For this review, take the finished solid that the model builds, in its own axes (mm). Coordinates: 2 decimals unless noted, no trailing zeros. Loops run counter-clockwise (first coordinate to the right, second up) from the corner with the lowest first, then second, coordinate; pieces in that order, holes last.
1. Take a section at A-A, the plane y = -70. State the section outline as (x, z) points, then the cut area to 3 significant figures.
2. Take a section at C-C, the plane y = 0. State the section outline as (x, z) points, then the cut area to 3 significant figures.
3. Take a section at D-D, the plane z = 4.2. State the section outline as (x, y) points, then the cut area to 3 significant figures.
4. To check wall thickness, follow probe 1 along Y at (x, z) = (40, 3.6); probe 2 along Y at (x, z) = (0, 3.8); probe 3 along X at (y, z) = (-48.5, 0.35). State the ranges of each line that lie inside material, in increasing order.
5. Clearance check with flat-ended pins moving along their axes: P1, Ø3, axis at x = 16.5, z = 2.5, coming from the +Y side; P2, Ø3, axis at x = 25.5, z = 1, coming from the +Y side; P3, Ø1, axis at y = 8.5, z = 3, coming from the -X side. State where each tip first meets the part, or that it passes through.
6. Take a section at B-B, the plane x = -40. State the section outline as (y, z) points.
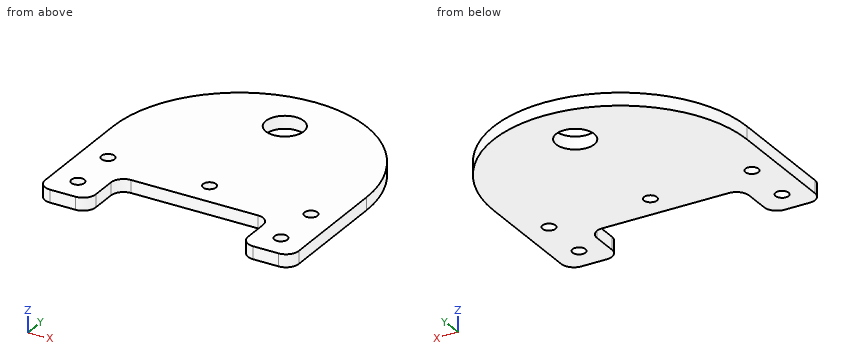
```python
from build123d import *

# Parameters (mm, degrees)
SKETCH_1_R      = 7.5
SKETCH_1_R_2    = 2.55
EXTRUDE_1_DEPTH = 5
SKETCH_2_W      = 20
SKETCH_2_H      = 20
SKETCH_2_R      = 2.55
EXTRUDE_2_DEPTH = 5
FILLET_1_R      = 5


with BuildPart() as part:
    # ｽｹｯﾁ1 → ﾎﾞｽ - 押し出し1 (new body)
    with BuildSketch(Plane.XY):
        with BuildLine():
            Line((-50, -60), (50, -60))
            Line((50, -60), (50, -30))
            ThreePointArc((50, -30), (0, 20), (-50, -30))
            Line((-50, -30), (-50, -60))
        make_face()
        Circle(SKETCH_1_R, mode=Mode.SUBTRACT)
        with Locations((-40, -50)):
            Circle(SKETCH_1_R_2, mode=Mode.SUBTRACT)
        with Locations((0, -50)):
            Circle(SKETCH_1_R_2, mode=Mode.SUBTRACT)
        with Locations((40, -50)):
            Circle(SKETCH_1_R_2, mode=Mode.SUBTRACT)
    extrude(amount=EXTRUDE_1_DEPTH)

    # ｽｹｯﾁ2 → ﾎﾞｽ - 押し出し2 (add)
    # profile 1 of 2: a face of its own
    with BuildSketch(Plane.XY.offset(5)):
        with Locations((-40, -70)):
            Rectangle(SKETCH_2_W, SKETCH_2_H)
        with Locations((-40, -70)):
            Circle(SKETCH_2_R, mode=Mode.SUBTRACT)
    # profile 2 of 2: a face of its own
    with BuildSketch(Plane.XY.offset(5)):
        with Locations((40, -70)):
            Rectangle(SKETCH_2_W, SKETCH_2_H)
        with Locations(Location((40, -70, 0), (0, 0, 180))):
            Circle(SKETCH_2_R, mode=Mode.SUBTRACT)
    extrude(amount=-EXTRUDE_2_DEPTH)

    # ﾌｨﾚｯﾄ1
    fillet_1_edges = [part.edges().sort_by_distance(p)[0] for p in [
        (-50, -80, 2.5),
        (-30, -60, 2.5),
        (-30, -80, 2.5),
        (30, -60, 2.5),
        (50, -80, 2.5),
        (30, -80, 2.5),
    ]]
    fillet(fillet_1_edges, radius=FILLET_1_R)


solid = part.part
```
Results list:
1. outline: (-50, 0) - (-42.55, 0) - (-42.55, 5) - (-50, 5) - close; (-37.45, 0) - (-30, 0) - (-30, 5) - (-37.45, 5) - close; (30, 0) - (37.45, 0) - (37.45, 5) - (30, 5) - close; (42.55, 0) - (50, 0) - (50, 5) - (42.55, 5) - close
1. area: 149 mm2
2. outline: (-40, 0) - (-7.5, 0) - (-7.5, 5) - (-40, 5) - close; (7.5, 0) - (40, 0) - (40, 5) - (7.5, 5) - close
2. area: 325 mm2
3. outline: (-50, -75) arc R5 ccw to (-45, -80) - (-35, -80) arc R5 ccw to (-30, -75) - (-30, -65) arc R5 cw to (-25, -60) - (25, -60) arc R5 cw to (30, -65) - (30, -75) arc R5 ccw to (35, -80) - (45, -80) arc R5 ccw to (50, -75) - (50, -30) arc R50 ccw to (-50, -30) - close; hole circle Ø5.1 at (-40, -70); hole circle Ø5.1 at (-40, -50); hole circle Ø15 at (0, 0); hole circle Ø5.1 at (0, -50); hole circle Ø5.1 at (40, -70); hole circle Ø5.1 at (40, -50)
3. area: 7,440 mm2
4. probe 1: y = -80 to -72.55, -67.45 to -52.55, -47.45 to 0
4. probe 2: y = -60 to -52.55, -47.45 to -7.5, 7.5 to 20
4. probe 3: x = -50 to -42.06, -37.94 to -2.06, 2.06 to 37.94, 42.06 to 50
5. P1: stops at y = 17.7
5. P2: stops at y = 13.86
5. P3: stops at x = -32.5
6. outline: (-80, 0) - (-72.55, 0) - (-72.55, 5) - (-80, 5) - close; (-67.45, 0) - (-52.55, 0) - (-52.55, 5) - (-67.45, 5) - close; (-47.45, 0) - (0, 0) - (0, 5) - (-47.45, 5) - close
